```python
from build123d import *

# Parameters (mm, degrees)
SKETCH1_R           = 2.75
SKETCH1_R_2         = 1.5
BOSS_EXTRUDE1_DEPTH = 8
BOSS_EXTRUDE2_START = -8
BOSS_EXTRUDE2_DEPTH = 8
CIRPATTERN2_COUNT   = 8
CUT_EXTRUDE1_DEPTH  = 10


with BuildPart() as part:
    # Sketch1 → Boss-Extrude1 (new body)
    with BuildSketch(Plane.XY):
        Circle(SKETCH1_R)
        Circle(SKETCH1_R_2, mode=Mode.SUBTRACT)
    extrude(amount=BOSS_EXTRUDE1_DEPTH)

    # Sketch3 → Boss-Extrude2 (add)
    with BuildSketch(Plane.XY.offset(8).offset(BOSS_EXTRUDE2_START)):
        with BuildLine():
            ThreePointArc((0.743305991, 2.647639742), (0, 2.75), (-0.743305991, 2.647639742))
            add(Edge.make_bspline(
                [(-0.271475541, 4.241320671), (-0.733052657, 3.513929186), (-0.743305991, 2.647639742)],
                knots=[0, 0, 0, 1, 1, 1], degree=2))
            ThreePointArc((-0.271475541, 4.241320671), (0, 4.25), (0.271475541, 4.241320671))
            add(Edge.make_bspline(
                [(0.271475541, 4.241320671), (0.733052657, 3.513929186), (0.743305991, 2.647639742)],
                knots=[0, 0, 0, 1, 1, 1], degree=2))
        make_face()
    boss_extrude2 = extrude(amount=BOSS_EXTRUDE2_DEPTH)

    # CirPattern2: Boss-Extrude2 ×8 about axis
    cirpattern2_axis = Axis((0, 0, 8), (0, 0, -1))
    for i in range(1, CIRPATTERN2_COUNT):
        add(boss_extrude2.rotate(cirpattern2_axis, i * 360 / CIRPATTERN2_COUNT))

    # Sketch4 → Cut-Extrude1 (cut)
    with BuildSketch(Plane.XY.offset(8)):
        with BuildLine():
            Line((-0.9, 2.224859546), (-0.9, 0.9))
            Line((-0.9, 0.9), (-2.224859546, 0.9))
            ThreePointArc((-2.224859546, 0.9), (-2.4, 0), (-2.224859546, -0.9))
            Line((-2.224859546, -0.9), (-0.9, -0.9))
            Line((-0.9, -0.9), (-0.9, -2.224859546))
            ThreePointArc((-0.9, -2.224859546), (0, -2.4), (0.9, -2.224859546))
            Line((0.9, -2.224859546), (0.9, -0.9))
            Line((0.9, -0.9), (2.224859546, -0.9))
            ThreePointArc((2.224859546, -0.9), (2.4, 0), (2.224859546, 0.9))
            Line((2.224859546, 0.9), (0.9, 0.9))
            Line((0.9, 0.9), (0.9, 2.224859546))
            ThreePointArc((0.9, 2.224859546), (0, 2.4), (-0.9, 2.224859546))
        make_face()
    extrude(amount=-CUT_EXTRUDE1_DEPTH, mode=Mode.SUBTRACT)


solid = part.part
```
The model under review builds one solid part; all positions refer to its coordinate system, in mm. A direction names the side the tool comes from. Coordinates: 2 decimals unless noted, no trailing zeros. Order: outer loops, then holes, each group sorted by start corner. A loop starts at its lowest first (then second) coordinate and runs counter-clockwise, first axis right, second up. Notation, with made-up numbers: (-23.75, 49) -> (-13.75, 49) arc R3 cw to (-13.75, 54) -> close; hole circle Ø9 at (16, 9). An arc over 180 degrees is marked (long way). Answer in a Markdown table with one row per item. Add a question column.
Item 1: We need section A-A on y = 0. Write out the cut boundary in (x, z).
Item 2: Machinability: for faces 1 (the cylindrical face through (2.4, 0, 4.1)), 2 (the flat face through (-1.3, -1.2, 8)), which of the approach directions +Z, -Z, +X, -X, +Y, -Y give a long, thin tool a straight path to every point of the face, cutting with its end or side? Answer none if there is none.
Item 3: To check wall thickness, follow probe 1 along Y at (x, z) = (-2.5, 5); probe 2 along X at (y, z) = (-0.25, 3). State the ranges of each line that lie inside material, in increasing order.
Item 4: Clearance check with flat-ended pins moving along their axes: pin 1 (2 mm diameter, centred on y = 2.5, z = 5, fed in from +X); pin 2 (0.5 mm diameter, centred on y = 1.5, z = 4.5, fed in from -X); pin 3 (1.1 mm diameter, centred on y = -1.5, z = 5, fed in from +X). State where each tip first meets the part, or that it passes through.
Item 5: Mouldability with a two-part tool opening along X and no side actions: class faces 3 (the flat face through (-1.3, -1.2, 0)), 4 (the flat face through (2, -0.9, 4)) as +X half, -X half, draft (parallel to the pull), parting line (faces both ways), or undercut.
Final values:
| question | item | result |
|---|---|---|
| 1 | outline | (-4.25, 0) -> (-2.4, 0) -> (-2.4, 8) -> (-4.25, 8) -> close; (2.4, 0) -> (4.25, 0) -> (4.25, 8) -> (2.4, 8) -> close |
| 2 | face 1 | +Z, -Z |
| 2 | face 2 | +Z, +X, -X, +Y, -Y |
| 3 | probe 1 | y = -3.11 to -1.46, -1.15 to 1.15, 1.46 to 3.11 |
| 3 | probe 2 | x = -4.24 to -2.39, 2.39 to 4.24 |
| 4 | pin 1 | stops at x = 3.19 |
| 4 | pin 2 | stops at x = -2.73 |
| 4 | pin 3 | stops at x = 2.91 |
| 5 | face 3 | draft |
| 5 | face 4 | undercut |
